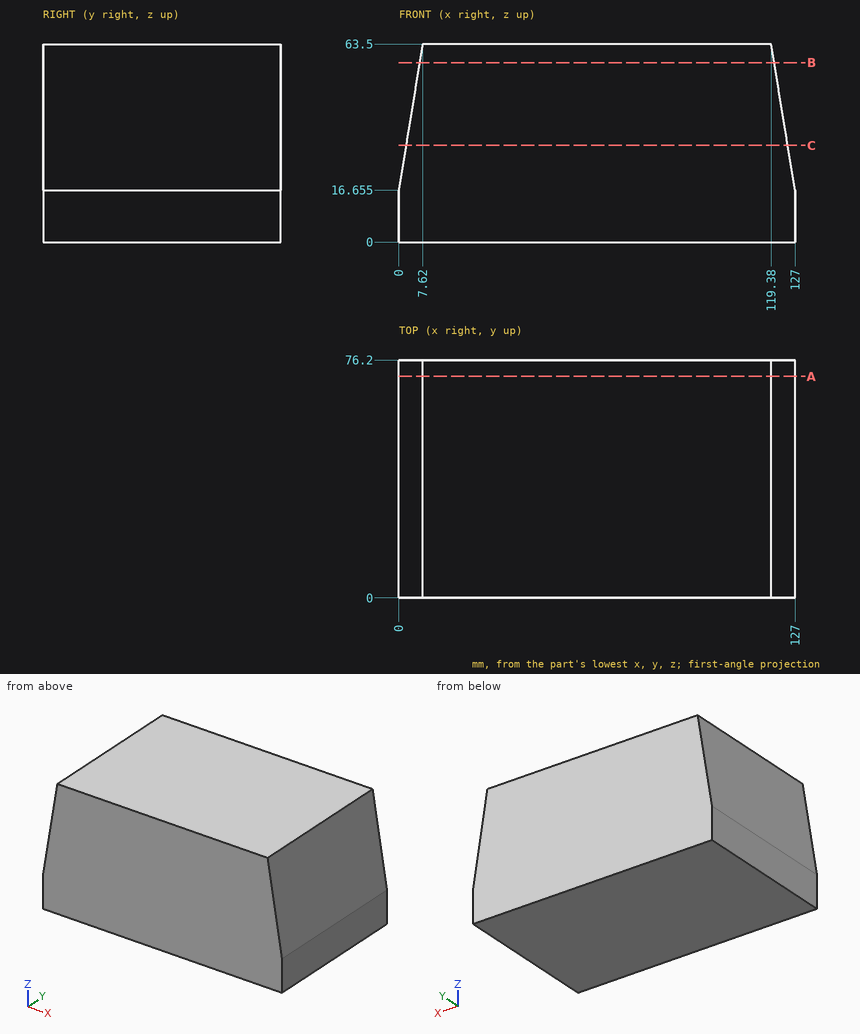
Geometry: see drawing. Coordinates: mm, zero at the bounding-box minimum. Round coordinates to 2 decimals unless told otherwise and drop trailing zeros. Order: outer loops, then holes, each group sorted by start corner. A loop starts at its lowest first (then second) coordinate and runs counter-clockwise, first axis right, second up. Notation, with made-up numbers: (7.5, -29) - (61.5, -29) arc R18 cw to (61.5, -22) - close; hole circle Ø9 at (-20, 6.25). An arc over 180 degrees is marked (long way). One line per question, with ' | ' between items. Start each with the question number.
1) Cut plane C-C, the plane z = 31. Return the cut outline in (x, y), then the cut area to 3 significant figures.
2) Contact query for flat-ended pins moving along their axis: P1, Ø6, axis at y = 34.5, z = 43.5, coming from the +X side; P2, Ø1, axis at y = 61, z = 31, coming from the +X side; P3, Ø12, axis at y = 13.5, z = 32.5, coming from the -X side. Output: stop coordinate, or through.
3) Cut plane A-A, the plane y = 71. Return the cut outline in (x, z) (1 decimal).
4) Cut plane B-B, the plane z = 57.5. Return the cut outline in (x, y), then the cut area to 4 significant figures.
5) Ray query, probe 1 along X at (y, z) = (21.5, 26.5); probe 2 along X at (y, z) = (13.5, 39.5). Return the intervals inside material, ascending.
Worked out:
1) outline: (2.33, 0) - (124.67, 0) - (124.67, 76.2) - (2.33, 76.2) - close | area: 9,320 mm^2
2) P1: stops at x = 123.12 | P2: stops at x = 124.75 | P3: stops at x = 1.6
3) outline: (0, 0) - (127, 0) - (127, 16.7) - (119.4, 63.5) - (7.6, 63.5) - (0, 16.7) - close
4) outline: (6.64, 0) - (120.36, 0) - (120.36, 76.2) - (6.64, 76.2) - close | area: 8,665 mm^2
5) probe 1: x = 1.6 to 125.4 | probe 2: x = 3.72 to 123.28
